Job drawing, mm, ordinate dimensions from the low corner. One solid piece. Coordinates: 2 decimals unless noted, no trailing zeros. Write each loop counter-clockwise with the first axis right and the second up, starting at its lowest first coordinate (ties: lowest second). Pieces come first, ordered by that corner, then holes. Notation, with made-up numbers: (79, 17.25) - (101, 17.25) arc R23 ccw to (101, 36.25) - close; hole circle Ø3 at (-31, -6.75). An arc over 180 degrees is marked (long way). Use a Markdown table: item, result.
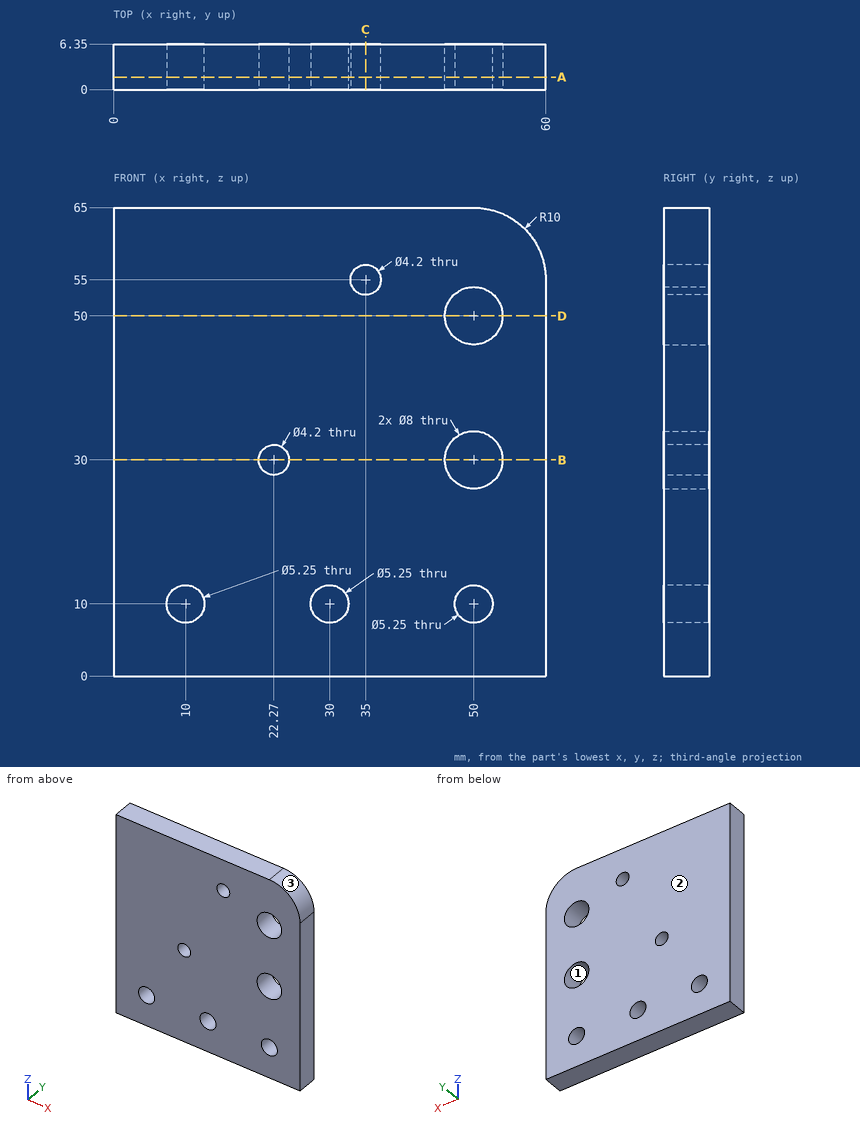
Item 1: Band-saw the part on B-B, the plane z = 30. Give the cut face in (x, y).
From the geometry:
| item | result |
|---|---|
| outline | (0, 0) - (20.17, 0) - (20.17, 6.35) - (0, 6.35) - close; (24.37, 0) - (46, 0) - (46, 6.35) - (24.37, 6.35) - close; (54, 0) - (60, 0) - (60, 6.35) - (54, 6.35) - close |
Item 2: Band-saw the part on A-A, the plane y = 1.75. Give the cut face in (x, z) (3 decimals).
From the geometry:
| item | result |
|---|---|
| outline | (0, 0) - (60, 0) - (60, 55) arc R10 ccw to (50, 65) - (0, 65) - close; hole circle Ø5.25 at (10, 10); hole circle Ø4.2 at (22.27, 30); hole circle Ø5.25 at (30, 10); hole circle Ø4.2 at (35, 55); hole circle Ø8 at (50, 30); hole circle Ø8 at (50, 50); hole circle Ø5.25 at (50, 10) |
Item 3: Drill centre lines: probe 1 along X at (y, z) = (4.5, 30); probe 2 along X at (y, z) = (3, 10) (3 decimals); probe 3 along Z at (x, y) = (50, 1.5) (3 decimals). Where is each one in solid material? Low to high.
From the geometry:
| item | result |
|---|---|
| probe 1 | 0 to 20.17, 24.37 to 46, 54 to 60 |
| probe 2 | 0 to 7.375, 12.625 to 27.375, 32.625 to 47.375, 52.625 to 60 |
| probe 3 | 0 to 7.375, 12.625 to 26, 34 to 46, 54 to 65 |
Item 4: Two-plate mould, pull along Z, no slides. Class the marked faces 1, 2 and 3: pulls with the +Z half, pulls with the -Z half, needs draft (parallel to the pull), parting line crosses it, or undercut.
From the geometry:
| item | result |
|---|---|
| face 1 | undercut |
| face 2 | needs draft |
| face 3 | pulls with the +Z half |
Item 5: Band-saw the part on C-C, the plane x = 35. Give the cut face in (y, z), then the cut area to 3 significant figures.
From the geometry:
| item | result |
|---|---|
| outline | (0, 0) - (6.35, 0) - (6.35, 52.9) - (0, 52.9) - close; (0, 57.1) - (6.35, 57.1) - (6.35, 65) - (0, 65) - close |
| area | 386 mm^2 |
Item 6: Band-saw the part on D-D, the plane z = 50. Give the cut face in (x, y).
From the geometry:
| item | result |
|---|---|
| outline | (0, 0) - (46, 0) - (46, 6.35) - (0, 6.35) - close; (54, 0) - (60, 0) - (60, 6.35) - (54, 6.35) - close |
Item 7: Drop flat-ended pins along their axis: P1, Ø3, axis at x = 23.5, z = 21.5, coming from the -Y side; P2, Ø4, axis at x = 50, z = 10, coming from the +Y side. Give the stop position or say it passes through.
From the geometry:
| item | result |
|---|---|
| P1 | y = 0 |
| P2 | through |
